Verification items for the finished model (mm, model axes). A direction names the side the tool comes from. Round coordinates to 2 decimals unless told otherwise and drop trailing zeros. Loops run counter-clockwise (first coordinate to the right, second up) from the corner with the lowest first, then second, coordinate; pieces in that order, holes last. Notation, with made-up numbers: (63, 57) -> (70, 57) arc R26 ccw to (70, 71) -> close; hole circle Ø10 at (-6, 47). An arc over 180 degrees is marked (long way). Use CSV: the item, a comma, the result in double quotes. Start each with the question number.
```python
from build123d import *

# Parameters (mm, degrees)
F0_R     = 2.75
F1_DEPTH = 5
F3_DEPTH = 60


with BuildPart() as f1:
    # F0 (on Top) → F1 (new body)
    with BuildSketch(Plane.XY):
        Polygon((74.1, 55.135), (-74.1, 55.135), (-90.235, 47.5), (-90.235, -47.5), (-74.1, -55.135), (74.1, -55.135), (90.235, -47.5), (90.235, 47.5), align=None)
        with Locations((-82.735, -40)):
            Circle(F0_R, mode=Mode.SUBTRACT)
        with Locations((82.735, -40)):
            Circle(F0_R, mode=Mode.SUBTRACT)
        with Locations((-82.735, 40)):
            Circle(F0_R, mode=Mode.SUBTRACT)
        with Locations((82.735, 40)):
            Circle(F0_R, mode=Mode.SUBTRACT)
    extrude(amount=F1_DEPTH)

    # F2 (on face) → F3 (join)
    with BuildSketch(Plane.XY.offset(5)):
        with BuildLine():
            ThreePointArc((74.1, 50.135), (72.635534, 53.670534), (69.1, 55.135))
            Line((69.1, 55.135), (-69.1, 55.135))
            ThreePointArc((-69.1, 55.135), (-72.635534, 53.670534), (-74.1, 50.135))
            Line((-74.1, 50.135), (-74.1, -50.135))
            ThreePointArc((-74.1, -50.135), (-72.635534, -53.670534), (-69.1, -55.135))
            Line((-69.1, -55.135), (69.1, -55.135))
            ThreePointArc((69.1, -55.135), (72.635534, -53.670534), (74.1, -50.135))
            Line((74.1, -50.135), (74.1, 50.135))
        make_face()
        Polygon((-5, 50.5), (0, 50.5), (5, 50.5), (5, 51.135), (25.1, 51.135), (25.1, 50.5), (35.1, 50.5), (35.1, 51.135), (50, 51.135), (50, 45), (71.1, 45), (71.1, -45), (50, -45), (50, -51.135), (35.1, -51.135), (35.1, -50.5), (25.1, -50.5), (25.1, -51.135), (5, -51.135), (5, -50.5), (0, -50.5), (-5, -50.5), (-5, -51.135), (-25.1, -51.135), (-25.1, -50.5), (-35.1, -50.5), (-35.1, -51.135), (-50, -51.135), (-50, -45), (-71.1, -45), (-71.1, 45), (-50, 45), (-50, 51.135), (-35.1, 51.135), (-35.1, 50.5), (-25.1, 50.5), (-25.1, 51.135), (-5, 51.135), align=None, mode=Mode.SUBTRACT)
    extrude(amount=F3_DEPTH)


solid = f1.part
```
Q1. Cross-section at D-D (x = -62.5). Record the boundary of the cut face in (y, z) (3 decimals), and give its area (3 significant figures).
Q2. Cross-section at B-B (x = 20.5). Record the boundary of the cut face in (y, z) (3 decimals).
Q3. Cross-section at C-C (y = -16). Record the boundary of the cut face in (x, z) (3 decimals).
Q4. Release check for a two-part mould opening along X. For faces 4 (the face through (-17, -53, 65)), 5 (the face through (-74.1, 1, 35)), 6 (the face through (-15, 51.135, 35)) record: +X half, -X half, draft (parallel to the pull), parting line (faces both ways), or undercut.
Q5. Thickness scan on L1, parallel to X at y = -30.5, z = 37; L2, parallel to Y at x = 4.5, z = 7 (3 decimals); L3, parallel to Y at x = 45, z = 28 (3 decimals). Record the ranges inside material, lowest first. Write a range as from..to.
Q6. Cross-section at A-A (y = -40). Record the boundary of the cut face in (x, z) (3 decimals), and give its area (3 significant figures).
Q7. Tool access check on faces 1 (the face through (-30, -50.5, 35)), 2 (the face through (1, 55.135, 32)), 3 (the face through (72.674, 53.631, 34.58)). Record the directions out of +Z, -Z, +X, -X, +Y, -Y that give a thin tool (end or side, any length) a straight path to the whole face; none if there is none.
Q8. Depth check by flat-ended pin: pin 1 Ø5 at (x, y) = (5, -43) entering from +Z; pin 2 Ø3 at (y, z) = (-16.5, 33.5) entering from -X; pin 3 Ø0.7 at (y, z) = (-50.5, 32) entering from +X. Enter the tip coordinate at first touch or a pass-through.
Answer list:
1,outline,"(-55.135, 0) -> (55.135, 0) -> (55.135, 65) -> (45, 65) -> (45, 5) -> (-45, 5) -> (-45, 65) -> (-55.135, 65) -> close"
1,area,"1,770 mm2"
2,outline,"(-55.135, 0) -> (55.135, 0) -> (55.135, 65) -> (51.135, 65) -> (51.135, 5) -> (-51.135, 5) -> (-51.135, 65) -> (-55.135, 65) -> close"
3,outline,"(-90.235, 0) -> (90.235, 0) -> (90.235, 5) -> (74.1, 5) -> (74.1, 65) -> (71.1, 65) -> (71.1, 5) -> (-71.1, 5) -> (-71.1, 65) -> (-74.1, 65) -> (-74.1, 5) -> (-90.235, 5) -> close"
4,face 4,"draft"
4,face 5,"-X half"
4,face 6,"undercut"
5,L1,"x = -74.1..-71.1, 71.1..74.1"
5,L2,"y = -55.135..-50.5, 50.5..55.135"
5,L3,"y = -55.135..-51.135, 51.135..55.135"
6,outline,"(-90.235, 0) -> (-85.485, 0) -> (-85.485, 5) -> (-90.235, 5) -> close; (-79.985, 0) -> (79.985, 0) -> (79.985, 5) -> (74.1, 5) -> (74.1, 65) -> (71.1, 65) -> (71.1, 5) -> (-71.1, 5) -> (-71.1, 65) -> (-74.1, 65) -> (-74.1, 5) -> (-79.985, 5) -> close; (85.485, 0) -> (90.235, 0) -> (90.235, 5) -> (85.485, 5) -> close"
6,area,"1,210 mm2"
7,face 1,"+Z"
7,face 2,"+Z, -Z, +X, -X, +Y"
7,face 3,"+Z, +X, +Y"
8,pin 1,"stops at z = 5"
8,pin 2,"stops at x = -74.1"
8,pin 3,"stops at x = 74.1"
